Geometry check sheet. Reference: drawing and pictorial views, mm from the part's lowest x, y, z. A direction names the side the tool comes from. Give positions to 0.01 mm unless a question says otherwise; leave off trailing zeros. Order: outer loops, then holes, each group sorted by start corner. A loop starts at its lowest first (then second) coordinate and runs counter-clockwise, first axis right, second up. Notation, with made-up numbers: (55, 15) -> (66, 15) arc R20 ccw to (66, 33) -> close; hole circle Ø5 at (-9, 7.5). An arc over 180 degrees is marked (long way). Write each question's results on one line, items separated by ' | '. Start each with the question number.
1. Set-up check for the marked faces 4, 5 and 6: record each of +Z, -Z, +X, -X, +Y, -Y from which the full face is reachable in a straight line by a thin tool's end or side.
2. Cross-section at C-C, the plane y = 2. Enter the section's corners in (x, z) (1 decimal).
3. Depth check by flat-ended pin: pin 1 Ø3 at (x, z) = (29, 4) entering from -Y; pin 2 Ø1 at (x, y) = (17, 1.5) entering from +Z. Enter the tip coordinate at first touch or a pass-through.
4. Mould release check, pull along X, two halves, no side actions. Record for the marked faces 1, 2 and 3: +X half, -X half, draft (parallel to the pull), parting line (faces both ways), or undercut.
5. Cross-section at A-A, the plane z = 14. Enter the section's corners in (x, y).
6. Cross-section at D-D, the plane x = 18. Enter the section's corners in (y, z).
7. Material ranges on L1, parallel to X at y = 0.55, z = 4; L2, parallel to X at y = 2.3, z = 10.75; L3, parallel to X at y = 1.7, z = 18.5 (1 decimal), recorded low to high. Write a range as from..to.
8. Cross-section at B-B, the plane y = 0.45. Enter the section's corners in (x, z) (1 decimal).
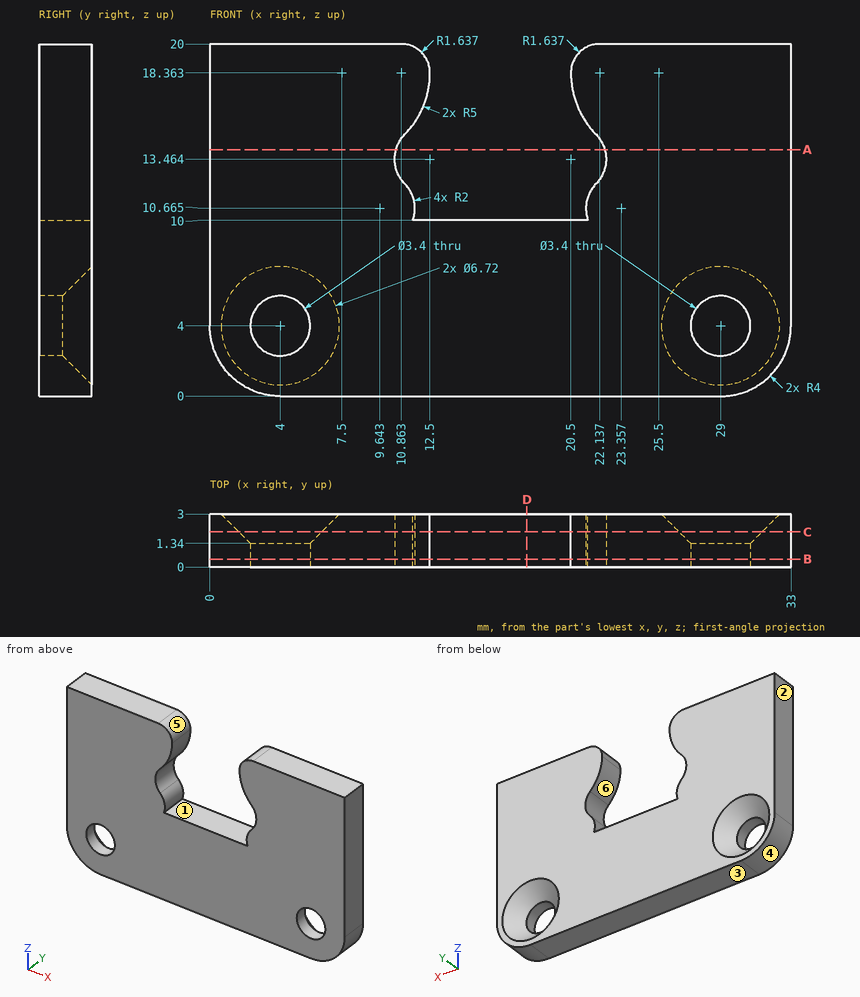
Results below:
1) face 4: -Z, -X, +Y, -Y | face 5: +Z, +Y, -Y | face 6: +Y, -Y
2) outline: (0, 4) arc R4 ccw to (4, 0) -> (29, 0) arc R4 ccw to (33, 4) -> (33, 20) -> (22.1, 20) arc R1.6 ccw to (20.5, 18.4) arc R5 ccw to (21.9, 14.9) arc R2 cw to (21.9, 12.1) arc R2 ccw to (21.5, 10) -> (11.5, 10) arc R2 ccw to (11.1, 12.1) arc R2 cw to (11.1, 14.9) arc R5 ccw to (12.5, 18.4) arc R1.6 ccw to (10.9, 20) -> (0, 20) -> close; hole circle Ø4.7 at (4, 4); hole circle Ø4.7 at (29, 4)
3) pin 1: passes through | pin 2: stops at z = 10
4) face 1: undercut | face 2: -X half | face 3: draft
5) outline: (0, 0) -> (10.57, 0) -> (10.57, 3) -> (0, 3) -> close; (22.43, 0) -> (33, 0) -> (33, 3) -> (22.43, 3) -> close
6) outline: (0, 0) -> (3, 0) -> (3, 10) -> (0, 10) -> close
7) L1: x = 0..2.3, 5.7..27.3, 30.7..33 | L2: x = 0..11.64, 21.36..33 | L3: x = 0..12.5, 20.5..33
8) outline: (0, 4) arc R4 ccw to (4, 0) -> (29, 0) arc R4 ccw to (33, 4) -> (33, 20) -> (22.1, 20) arc R1.6 ccw to (20.5, 18.4) arc R5 ccw to (21.9, 14.9) arc R2 cw to (21.9, 12.1) arc R2 ccw to (21.5, 10) -> (11.5, 10) arc R2 ccw to (11.1, 12.1) arc R2 cw to (11.1, 14.9) arc R5 ccw to (12.5, 18.4) arc R1.6 ccw to (10.9, 20) -> (0, 20) -> close; hole circle Ø3.4 at (4, 4); hole circle Ø3.4 at (29, 4)
